Autodesk Inventor part; units mm, degrees
ref_plane "YZ Plane" through (0, 0, 0) normal (1, 0, 0) x (0, 1, 0)
ref_plane "XZ Plane" through (0, 0, 0) normal (0, 1, 0) x (-1, 0, 0)
ref_plane "XY Plane" through (0, 0, 0) normal (0, 0, 1) x (1, 0, 0)
sketch "Sketch_1" plane through (0, 0, 0) normal (1, 0, 0) x (0, 1, 0)
  line L0 (0, 20) -> (0, 0)
  line L1 (0, 0) -> (20, 0)
  line L2 (20, 0) -> (20, 3)
  line L3 (20, 3) -> (3, 20)
  line L4 (3, 20) -> (0, 20)
extrude "Extrusion1" add sketch "Sketch_1" along normal mid plane 17
sketch "Sketch_2" plane through (0, 0, 0) normal (1, 0, 0) x (0, 1, 0)
  line L0 (3, 20) -> (3, 3.5)
  arc A0 (3, 3.5) -> (3.5, 3) centre (3.5, 3.5) ccw
  line L1 (3.5, 3) -> (20, 3)
  line L2 (20, 3) -> (3, 20)
extrude "Extrusion2" cut sketch "Sketch_2" along normal mid plane 13
sketch "Sketch_3" plane through (0, 0, 0) normal (1, 0, 0) x (0, 1, 0)
  line L0 (0, 3) -> (0, 0)
  line L1 (0, 0) -> (3, 0)
  line L2 (3, 0) -> (3, 1)
  line L3 (3, 1) -> (1, 1)
  line L4 (1, 1) -> (1, 3)
  line L5 (1, 3) -> (0, 3)
extrude "Extrusion3" cut sketch "Sketch_3" along normal mid plane 12
sketch "Sketch_4" plane through (0, 0, 0) normal (1, 0, 0) x (0, 1, 0)
  line L0 (0, 19) -> (0, 16)
  line L1 (0, 16) -> (1, 16)
  line L2 (1, 16) -> (1, 19)
  line L3 (1, 19) -> (0, 19)
extrude "Extrusion4" cut sketch "Sketch_4" along normal mid plane 12
sketch "Sketch_5" plane through (0, 0, 0) normal (1, 0, 0) x (0, 1, 0)
  line L0 (16, 1) -> (16, 0)
  line L1 (16, 0) -> (19, 0)
  line L2 (19, 0) -> (19, 1)
  line L3 (19, 1) -> (16, 1)
extrude "Extrusion5" cut sketch "Sketch_5" along normal mid plane 12
sketch "Sketch_10" plane through (0, 0, 0) normal (0, 1, 0) x (-1, 0, 0)
  line L0 (2.75, 8) -> (2.75, 11)
  arc A0 (2.75, 11) -> (-2.75, 11) centre (0, 11) ccw
  line L1 (-2.75, 11) -> (-2.75, 8)
  arc A1 (-2.75, 8) -> (2.75, 8) centre (0, 8) ccw
extrude "Extrusion6" cut sketch "Sketch_10" along normal blind 5
sketch "Sketch_11" plane through (0, 0, 0) normal (0, 0, 1) x (1, 0, 0)
  arc A0 (-2.75, 8) -> (2.75, 8) centre (0, 8) ccw
  line L0 (2.75, 8) -> (2.75, 11)
  arc A1 (2.75, 11) -> (-2.75, 11) centre (0, 11) ccw
  line L1 (-2.75, 11) -> (-2.75, 8)
extrude "Extrusion7" cut sketch "Sketch_11" along normal blind 5
properties part number "14056_m"
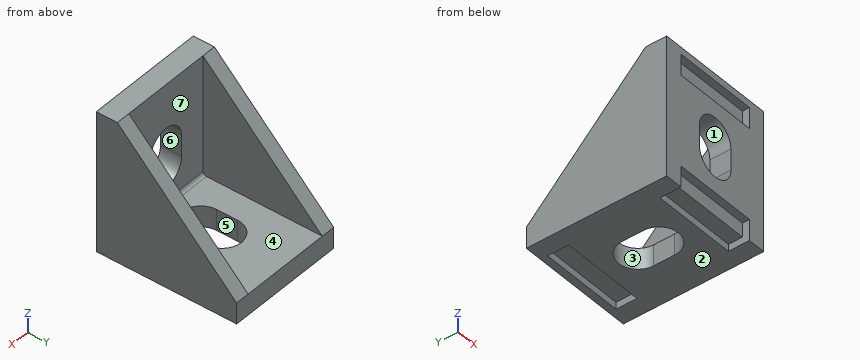
Geometry check sheet. Reference: the model listing, model coordinates, mm. Face numbers are marked on the shaded views. A direction names the side the tool comes from. Round coordinates to 2 decimals unless told otherwise and drop trailing zeros. Loops run counter-clockwise (first coordinate to the right, second up) from the corner with the lowest first, then second, coordinate; pieces in that order, holes last. Notation, with made-up numbers: (38.5, 51.25) - (64.5, 51.25) arc R23 ccw to (64.5, 85.25) - close; hole circle Ø7 at (-0.75, 1). An arc over 180 degrees is marked (long way). Write item = value, one per line. Start each with the question number.
1. Thickness scan on line 1 (X direction, y = 7.5, z = 5.5); line 2 (Z direction, x = 3.5, y = 12.75); line 3 (Z direction, x = 4.25, y = 16.25). Record the ranges inside material, lowest first.
2. Section check C-C on z = 17. Enter the section's corners in (x, y), then the cut area to 3 significant figures.
3. Set-up check for the marked faces 5, 6 and 7: record each of +Z, -Z, +X, -X, +Y, -Y from which the full face is reachable in a straight line by a thin tool's end or side.
4. Depth check by flat-ended pin: pin 1 (6 mm diameter, centred on y = 10.5, z = 17.5, fed in from -X); pin 2 (0.5 mm diameter, centred on x = 0.5, y = 0.5, fed in from -Z); pin 3 (0.8 mm diameter, centred on x = 1, z = 0.5, fed in from -Y); pin 4 (1.1 mm diameter, centred on x = 2, z = 0.5, fed in from -Y). Enter the tip coordinate at first touch or a pass-through.
5. Section check A-A on z = 8.5. Enter the section's corners in (x, y).
6. Section check D-D on y = 4.5. Enter the section's corners in (x, z), then the cut area to 3 significant figures.
7. Section check B-B on x = 0. Enter the section's corners in (y, z), then the cut area to 3 significant figures.
8. Mould release check, pull along Z, two halves, no side actions. Record for the marked faces 1, 2, 3 and 4: released by +Z, released by -Z, zero draft, split by the parting line, or undercut.
Working result:
q1.line_1 = -8.5 to -6.5, 6.5 to 8.5
q1.line_2 = 0 to 3
q1.line_3 = 1 to 3
q2.outline = (-8.5, 0) - (-6, 0) - (-6, 1) - (6, 1) - (6, 0) - (8.5, 0) - (8.5, 6) - (6.5, 6) - (6.5, 3) - (-6.5, 3) - (-6.5, 6) - (-8.5, 6) - close
q2.area = 51.0 mm^2
q3.face_5 = +Z, -Z
q3.face_6 = +Y, -Y
q3.face_7 = +Z, +Y
q4.pin_1 = through
q4.pin_2 = 3
q4.pin_3 = 3
q4.pin_4 = 1
q5.outline = (-8.5, 0) - (-2.75, 0) - (-2.75, 3) - (-6.5, 3) - (-6.5, 14.5) - (-8.5, 14.5) - close; (2.75, 0) - (8.5, 0) - (8.5, 14.5) - (6.5, 14.5) - (6.5, 3) - (2.75, 3) - close
q6.outline = (-8.5, 0) - (8.5, 0) - (8.5, 18.5) - (6.5, 18.5) - (6.5, 3) - (-6.5, 3) - (-6.5, 18.5) - (-8.5, 18.5) - close
q6.area = 113 mm^2
q7.outline = (0, 3) - (1, 3) - (1, 1) - (3, 1) - (3, 0) - (5.25, 0) - (5.25, 3) - (3.5, 3) arc R0.5 cw to (3, 3.5) - (3, 5.25) - (0, 5.25) - close; (0, 13.75) - (3, 13.75) - (3, 20) - (0, 20) - (0, 19) - (1, 19) - (1, 16) - (0, 16) - close; (13.75, 0) - (16, 0) - (16, 1) - (19, 1) - (19, 0) - (20, 0) - (20, 3) - (13.75, 3) - close
q7.area = 49.1 mm^2
q8.face_1 = undercut
q8.face_2 = released by -Z
q8.face_3 = zero draft
q8.face_4 = released by +Z
